Geometry: final body of the model. Coordinates: model frame, mm. Face numbers are marked on the shaded views. A direction names the side the tool comes from. Coordinates: 2 decimals unless noted, no trailing zeros. Order: outer loops, then holes, each group sorted by start corner. A loop starts at its lowest first (then second) coordinate and runs counter-clockwise, first axis right, second up. Notation, with made-up numbers: (18, -19.5) - (32, -19.5) arc R31 cw to (32, 18.5) - close; hole circle Ø3 at (87.25, -26). An arc over 180 degrees is marked (long way). Use a Markdown table: item, result. Add a question column.
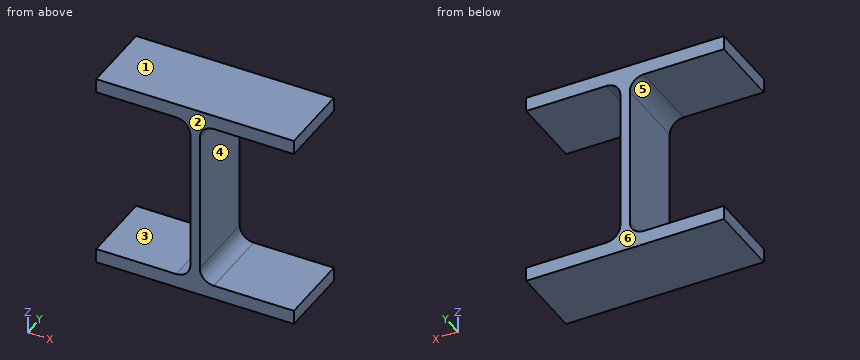
Solid Edge part; units mm, degrees
sketch "Sketch1" plane through (0, 0, 0) normal (0, -1, 0) x (1, 0, 0)
  line L0 (63.5, 63.627) -> (-63.5, 63.627)
  line L1 (-63.5, 63.627) -> (-63.5, 54.483)
  line L2 (-63.5, 54.483) -> (-12.0332, 54.483)
  arc A0 (-12.0332, 54.483) -> (-3.048, 45.4977) centre (-12.0332, 45.4977) cw
  line L3 (-3.048, 45.4977) -> (-3.048, -45.4977)
  arc A1 (-3.048, -45.4977) -> (-12.0332, -54.483) centre (-12.0332, -45.4977) cw
  line L4 (-12.0332, -54.483) -> (-63.5, -54.483)
  line L5 (-63.5, -54.483) -> (-63.5, -63.627)
  line L6 (-63.5, -63.627) -> (63.5, -63.627)
  line L7 (63.5, -54.483) -> (63.5, -63.627)
  line L8 (12.0332, -54.483) -> (63.5, -54.483)
  arc A2 (3.048, -45.4977) -> (12.0332, -54.483) centre (12.0332, -45.4977) ccw
  line L9 (3.048, 45.4977) -> (3.048, -45.4977)
  arc A3 (12.0332, 54.483) -> (3.048, 45.4977) centre (12.0332, 45.4977) ccw
  line L10 (63.5, 54.483) -> (12.0332, 54.483)
  line L11 (63.5, 63.627) -> (63.5, 54.483)
extrude "Protrusion1" add sketch "Sketch1" against normal blind 47.625
1) Pin query (flat end, axial travel): pin 1 (14.5 mm diameter, centred on y = 18.5, z = 9, fed in from -X); pin 2 (1.5 mm diameter, centred on y = 8, z = -12.5, fed in from +X). Return the tip coordinate at first contact, or that it passes through.
2) Section C-C (z = -14.5). Return loops of the section in (x, y) (3 decimals), then the cut area to 3 significant figures.
3) Draft query along Z for the marked faces 1, 2 and 3. Return one class per face: pulls with the +Z half, pulls with the -Z half, needs draft (parallel to the pull), parting line crosses it, or undercut.
4) Ray query, line 1 along Z through (x, y) = (-40.5, 31.5); line 2 along X through (y, z) = (5, -15.5); line 3 along Z through (x, y) = (-5, 38.5). Return the intervals inside material, ascending.
5) Set-up query: the marked faces 4, 5 and 6. Return all of +Z, -Z, +X, -X, +Y, -Y with unobstructed straight access to the full face (end or side cutting, diameter ignored); none if empty.
6) Section A-A (x = 21). Return loops of the section in (y, z) (3 decimals).
7) Section B-B (y = 26.5). Return loops of the section in (x, z), then the cut area to 3 significant figures.
Values follow:
| question | item | result |
|---|---|---|
| 1 | pin 1 | stops at x = -3.05 |
| 1 | pin 2 | stops at x = 3.05 |
| 2 | outline | (-3.048, 0) - (3.048, 0) - (3.048, 47.625) - (-3.048, 47.625) - close |
| 2 | area | 290 mm² |
| 3 | face 1 | pulls with the +Z half |
| 3 | face 2 | needs draft |
| 3 | face 3 | undercut |
| 4 | line 1 | z = -63.63 to -54.48, 54.48 to 63.63 |
| 4 | line 2 | x = -3.05 to 3.05 |
| 4 | line 3 | z = -63.63 to -51.09, 51.09 to 63.63 |
| 5 | face 4 | +X, +Y, -Y |
| 5 | face 5 | -X, +Y, -Y |
| 5 | face 6 | +Z, -Z, +X, -X, +Y |
| 6 | outline | (0, -63.627) - (47.625, -63.627) - (47.625, -54.483) - (0, -54.483) - close; (0, 54.483) - (47.625, 54.483) - (47.625, 63.627) - (0, 63.627) - close |
| 7 | outline | (-63.5, -63.63) - (63.5, -63.63) - (63.5, -54.48) - (12.03, -54.48) arc R8.99 cw to (3.05, -45.5) - (3.05, 45.5) arc R8.99 cw to (12.03, 54.48) - (63.5, 54.48) - (63.5, 63.63) - (-63.5, 63.63) - (-63.5, 54.48) - (-12.03, 54.48) arc R8.99 cw to (-3.05, 45.5) - (-3.05, -45.5) arc R8.99 cw to (-12.03, -54.48) - (-63.5, -54.48) - close |
| 7 | area | 3,060 mm² |
